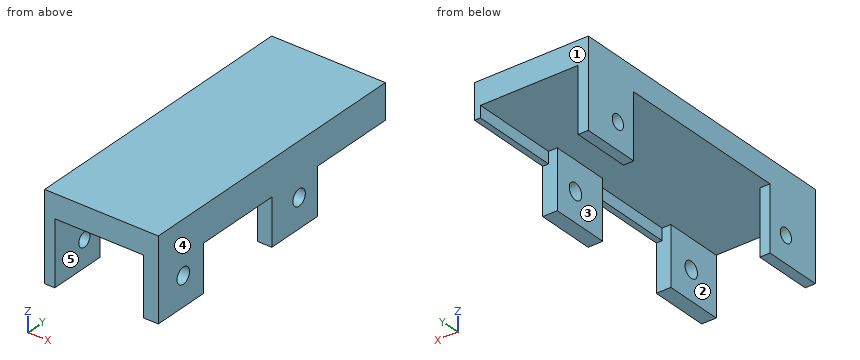
Autodesk Inventor part; units mm, degrees
ref_plane "YZ Plane" through (0, 0, 0) normal (1, 0, 0) x (0, 1, 0)
ref_plane "XZ Plane" through (0, 0, 0) normal (0, 1, 0) x (-1, 0, 0)
ref_plane "XY Plane" through (0, 0, 0) normal (0, 0, 1) x (1, 0, 0)
sketch "Skizze1" plane through (0, 0, 0) normal (0, 1, 0) x (-1, 0, 0)
  line L0 (0, 0) -> (0, 8)
  line L1 (0, 8) -> (2, 8)
  line L2 (2, 8) -> (2, 4)
  line L3 (2, 4) -> (39, 4)
  line L4 (39, 4) -> (39, 0)
  line L5 (0, 0) -> (13.2064, 0)
  line L6 (0, 0) -> (0, -8)
  line L7 (0, -8) -> (2, -8)
  line L8 (2, -8) -> (2, -4)
  line L9 (2, -4) -> (39, -4)
  line L10 (39, -4) -> (39, 0)
  dimension "d1" = 8
  dimension "d2" = 2
  dimension "d3" = 4
  dimension "d4" = 37
extrude "Extrusion1" add sketch "Skizze1" along normal mid plane 100
sketch "Skizze5" plane through (-39, -50, 4) normal (0, 0, 1) x (1, 0, 0)
  line L0 (0, 0) -> (0, 100)
  line L1 (0, 0) -> (3.5, 0)
  line L2 (3.5, 0) -> (3.5, 20)
  line L3 (3.5, 20) -> (0, 20)
  line L4 (0, 20) -> (0, 0)
  point P0 (39, 50)
  point P1 (0, 20.0912)
  dimension "d22" = 3.5
  dimension "d23" = 20
extrude "Extrusion3" add sketch "Skizze5" along normal blind 20 and the other way blind 30
sketch "Skizze6" plane through (-39, 50, 4) normal (0, 0, 1) x (1, 0, 0)
  line L0 (0, -80) -> (0, 0)
  line L1 (0, 0) -> (3.5, 0)
  line L2 (3.5, 0) -> (3.5, -20)
  line L3 (3.5, -20) -> (0, -20)
  line L4 (0, -20) -> (0, 0)
  point P0 (39, -50)
  point P1 (0, -19.9088)
  point P2 (0, -20)
  dimension "d26" = 20
  dimension "d32" = 3.5
extrude "Extrusion4" add sketch "Skizze6" along normal blind 20 and the other way blind 30
sketch "Esquisse11" plane through (-35.5, 30, -4) normal (1, 0, 0) x (0, 0, -1)
  line L0 (22, 20) -> (0, 20)
  line L1 (22, 20) -> (22, 0)
  line L2 (22, -60) -> (22, -80)
  point P0 (-4, -30)
  point P1 (13, 7)
  point P2 (13, -67)
  dimension "d57" = 13
  dimension "d58" = 74
  dimension "d59" = 9
  dimension "d60" = 9
hole "Perçage3" at (-35.5, 37, -17) at (-35.5, -37, -17) direction (-1, 0, 0) diameter 4.917 end through all
sketch "Esquisse21" plane through (-35.5, -50, 4) normal (1, 0, 0) x (0, 0, -1)
  line L0 (0, 100) -> (0, 80)
  line L1 (0, 20) -> (0, 80)
  line L2 (0, 20) -> (0, 0)
  line L3 (0, 100) -> (0, 0)
  line L4 (-36.3372, 0) -> (0, 0)
  line L5 (0, 0) -> (0, 115.7943)
  line L6 (0, 115.7943) -> (-36.3372, 115.7943)
  line L7 (-36.3372, 115.7943) -> (-36.3372, 0)
  point P0 (4, 50)
  point P1 (0, 20)
extrude "Extrusion15" cut sketch "Esquisse21" along normal mid plane 9999
sketch "Esquisse22" plane through (-2, -50, -4) normal (0, 0, -1) x (-1, 0, 0)
  line L0 (37, 15.4585) -> (37, 10.5415)
  line L1 (33.5, 10.5415) -> (33.5, 15.4585)
  line L2 (-2, 0) -> (3, 0)
  line L3 (3, 0) -> (3, 20)
  line L4 (3, 20) -> (-2, 20)
  line L5 (-2, 20) -> (-2, 0)
  line L6 (33.5, 0) -> (0, 0)
  line L7 (-2, 0) -> (-2, 100)
  point P0 (-2, 50)
  point P1 (0.5, 0)
  dimension "d92" = 5
  dimension "d93" = 0
  dimension "d94" = 0
extrude "Extrusion16" add sketch "Esquisse22" along normal blind 20
sketch "Esquisse23" plane through (-5, -50, -4) normal (-1, 0, 0) x (0, 0, 1)
  line L0 (0, 20) -> (-20, 20)
  line L1 (-20, 0) -> (-20, 20)
  point P0 (4, 50)
  point P1 (-10, 11)
  dimension "d104" = 9
  dimension "d105" = 10
hole "Perçage5" at (-5, -39, -14) direction (1, 0, 0) diameter 5.5 end through all
sketch "Esquisse24" plane through (-35.5, -30, -4) normal (0, 0, -1) x (-1, 0, 0)
  line L0 (-35.5, 0) -> (-35.5, 80)
  line L1 (-35.5, 50) -> (-30.5, 50)
  line L2 (-30.5, 50) -> (-30.5, 30)
  line L3 (-30.5, 30) -> (-35.5, 30)
  line L4 (-35.5, 30) -> (-35.5, 50)
  line L5 (-30.5, 0) -> (-35.5, 0)
  point P0 (-35.5, 30)
  dimension "d106" = 5
  dimension "d107" = 20
  dimension "d108" = 30
extrude "Extrusion17" add sketch "Esquisse24" along normal blind 20
sketch "Esquisse25" plane through (-5, 0, -4) normal (-1, 0, 0) x (0, 0, 1)
  line L0 (-20, 0) -> (-20, 20)
  line L1 (0, 20) -> (-20, 20)
  point P0 (4, 0)
  point P1 (-10, 12)
  dimension "d118" = 10
  dimension "d119" = 8
hole "Perçage6" at (-5, 12, -14) direction (1, 0, 0) diameter 5.5 end through all
properties part number "Befestigung Bremssattel"
Model file for the job. Use its own axes, mm. Face numbers are marked on the shaded views. A direction names the side the tool comes from. Coordinates: 2 decimals unless noted, no trailing zeros. Loops run counter-clockwise (first coordinate to the right, second up) from the corner with the lowest first, then second, coordinate; pieces in that order, holes last. Notation, with made-up numbers: M 11,-14.75 L 45,-14.75 A9 cw 45,-6.75 Z; hole C 72.5,71.5 d3. An arc over 180 degrees is marked long. Use CSV: the item, a comma, the result in double quotes. Start each with the question number.
1. Probe probe 1 along Y at (x, z) = (-1.55, -14); probe 2 along Y at (x, z) = (-36.35, -17); probe 3 along Z at (x, y) = (-3.15, -39). List the from-to ranges inside material, lowest first. Write a range as [from, to].
2. Band-saw the part on C-C, the plane x = -37. List the corners of the cut face in (y, z), then the cut area to 3 significant figures.
3. Flat gauge pins, fed straight in: pin 1 (2 mm diameter, centred on x = -1, y = 41.5, fed in from -Z); pin 2 (3 mm diameter, centred on y = -37, z = -17, fed in from -X); pin 3 (1.5 mm diameter, centred on x = -3, z = -12.5, fed in from +Y). Where does each tip first touch, or does it go through?
4. Two-plate mould, pull along X, no slides. Class the marked faces 1, 2 and 3: pulls with the +X half, pulls with the -X half, needs draft (parallel to the pull), parting line crosses it, or undercut.
5. Band-saw the part on D-D, the plane z = -12.5. List the corners of the cut face in (x, y), then the cut area to 3 significant figures.
6. Band-saw the part on A-A, the plane y = 12. List the corners of the cut face in (x, z).
7. Tool access for the marked faces 4 and 5: list every direction of +Z, -Z, +X, -X, +Y, -Y with a clear straight run to the whole face (end or side of a thin tool).
8. Band-saw the part on B-B, the plane z = -21.75. List the corners of the cut face in (x, y).
Entries:
1,probe 1,"y = [-50, -41.75], [-36.25, -30], [0, 9.25], [14.75, 20]"
1,probe 2,"y = [-50, -39.46], [-34.54, -30], [30, 34.54], [39.46, 50]"
1,probe 3,"z = [-24, -16.75], [-11.25, 4]"
2,outline,"M -50,-26 L -30,-26 L -30,-4 L 30,-4 L 30,-26 L 50,-26 L 50,4 L -50,4 Z; hole C -37,-17 d4.92; hole C 37,-17 d4.92"
2,area,"1,640 mm2"
3,pin 1,"stops at z = -8"
3,pin 2,"stops at x = -5"
3,pin 3,"stops at y = 20"
4,face 1,"needs draft"
4,face 2,"undercut"
4,face 3,"pulls with the -X half"
5,outline,"M -39,-50 L -35.5,-50 L -35.5,-30 L -39,-30 Z; M -39,30 L -35.5,30 L -35.5,50 L -39,50 Z; M -5,-50 L 0,-50 L 0,-41.3 L -5,-41.3 Z; M -5,-36.7 L 0,-36.7 L 0,-30 L -5,-30 Z; M -5,0 L 0,0 L 0,9.7 L -5,9.7 Z; M -5,14.3 L 0,14.3 L 0,20 L -5,20 Z"
5,area,"294 mm2"
6,outline,"M -39,-4 L -5,-4 L -5,-11.25 L 0,-11.25 L 0,4 L -39,4 Z; M -5,-24 L 0,-24 L 0,-16.75 L -5,-16.75 Z"
7,face 4,"+Z, -Z, +X, +Y, -Y"
7,face 5,"-Z, +Y, -Y"
8,outline,"M -39,-50 L -35.5,-50 L -35.5,-30 L -39,-30 Z; M -39,30 L -35.5,30 L -35.5,50 L -39,50 Z; M -5,-50 L 0,-50 L 0,-30 L -5,-30 Z; M -5,0 L 0,0 L 0,20 L -5,20 Z"
